from build123d import *

# Parameters (mm, degrees)
SKETCH1_R           = 1.85
SKETCH1_R_2         = 4
BOSS_EXTRUDE1_DEPTH = 2
CUT_EXTRUDE1_DEPTH  = 3


with BuildPart() as part:
    # Sketch1 → Boss-Extrude1 (new body)
    with BuildSketch(Plane(origin=(0, 0, 0), x_dir=(1, 0, 0), z_dir=(0, 1, 0))):
        with BuildLine():
            Line((39.272536472, 22.976935119), (-24.727463528, 22.976935119))
            ThreePointArc((-24.727463528, 22.976935119), (-38.227463528, 9.476935119), (-24.727463528, -4.023064881))
            Line((-24.727463528, -4.023064881), (39.272536472, -4.023064881))
            ThreePointArc((39.272536472, -4.023064881), (52.772536472, 9.476935119), (39.272536472, 22.976935119))
        make_face()
        with Locations((-24.727463528, 17.476935119)):
            Circle(SKETCH1_R, mode=Mode.SUBTRACT)
        with Locations((-24.727463528, 9.476935119)):
            Circle(SKETCH1_R_2, mode=Mode.SUBTRACT)
        with Locations((-32.727463528, 9.476935119)):
            Circle(SKETCH1_R, mode=Mode.SUBTRACT)
        with Locations((-24.727463528, 1.476935119)):
            Circle(SKETCH1_R, mode=Mode.SUBTRACT)
        with Locations((-16.727463528, 9.476935119)):
            Circle(SKETCH1_R, mode=Mode.SUBTRACT)
        with Locations((39.272536472, 17.476935119)):
            Circle(SKETCH1_R, mode=Mode.SUBTRACT)
        with Locations((39.272536472, 9.476935119)):
            Circle(SKETCH1_R_2, mode=Mode.SUBTRACT)
        with Locations((31.272536472, 9.476935119)):
            Circle(SKETCH1_R, mode=Mode.SUBTRACT)
        with Locations((47.272536472, 9.476935119)):
            Circle(SKETCH1_R, mode=Mode.SUBTRACT)
        with Locations((39.272536472, 1.476935119)):
            Circle(SKETCH1_R, mode=Mode.SUBTRACT)
    extrude(amount=BOSS_EXTRUDE1_DEPTH)

    # Sketch2 → Cut-Extrude1 (cut, through all)
    with BuildSketch(Plane(origin=(0, 2, 0), x_dir=(1, 0, 0), z_dir=(0, 1, 0))):
        with BuildLine():
            Line((-23.067485442, 22.976935119), (42.777422328, 34.888708749))
            Line((42.777422328, 34.888708749), (45.278061915, 21.567578781))
            ThreePointArc((45.278061915, 21.567578781), (10.860216356, 10.387702722), (-23.067485442, 22.976935119))
        make_face()
        with BuildLine():
            Line((48.61621824, 19.220938968), (77.215135597, 13.399575669))
            Line((77.215135597, 13.399575669), (46.358944508, -30.129693903))
            Line((46.358944508, -30.129693903), (-23.067485442, -4.023064881))
            ThreePointArc((-23.067485442, -4.023064881), (14.611544165, 1.933144375), (48.61621824, 19.220938968))
        make_face()
    extrude(amount=-CUT_EXTRUDE1_DEPTH, mode=Mode.SUBTRACT)


solid = part.part
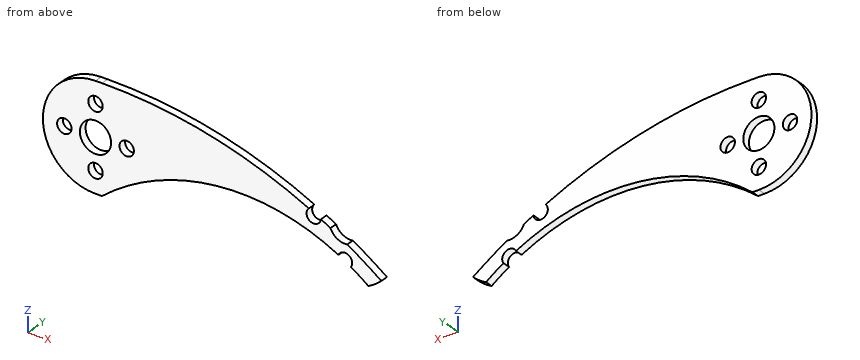
Can you work these out from the model? Positions are in its coordinate system, mm. Give positions to 0.01 mm unless a question says otherwise; leave off trailing zeros. Write each loop counter-clockwise with the first axis right and the second up, starting at its lowest first coordinate (ties: lowest second). Pieces come first, ordered by that corner, then holes. Notation, with made-up numbers: (17, -8) -> (21, -8) arc R22 cw to (21, 6) -> close; hole circle Ø8 at (62.25, -33.5). An arc over 180 degrees is marked (long way). Answer as a JSON object with one key per item and string values. Group by question number.
Item 1: Please list where these lines run through material, in increasing order: line 1 (Z direction, x = -24.5, y = 1.55); line 2 (X direction, y = 1.2, z = -18.75); line 3 (X direction, y = 1.65, z = -16.5). Write a range as [from, to].
Item 2: Suppose I cut it at A-A (y = 0.4). Please give me the cut outline in (x, z), plus the area to 3 significant figures.
Item 3: Suppose I cut it at C-C (x = 38.5). Please give me the cut outline in (y, z).
Item 4: I'm going to push a flat-ended pin straight in: P1, Ø1, axis at y = 1.5, z = -19.5, coming from the -X side. Where does the tip first touch, or does it pass through?
Item 5: Suppose I cut it at B-B (z = 2.5). Please give me the cut outline in (x, y).
Findings:
{
 "1": {"line 1": "z = [-22.98, -19.31], [-15.64, -13.47], [-5.48, -3.31], [0.36, 4.02]", "line 2": "x = [-34.54, -26.07], [-23.39, -17.2], [41.19, 47.96]", "line 3": "x = [-36.26, -26.3], [-23.16, -13.25], [37.24, 37.7], [40.84, 44.7]"},
 "2": {"outline": "(-24.73, -22.98) -> (-23.07, -22.98) arc R55.08 cw to (37.6, -16.69) arc R1.85 cw (long way) to (40.81, -18.51) arc R55.08 cw to (45.28, -21.57) arc R13.5 ccw to (48.62, -19.22) arc R122.16 ccw to (39.86, -13.43) arc R4 cw to (35.56, -10.96) arc R122.16 ccw to (33.11, -9.66) arc R1.85 cw (long way) to (30.02, -8.12) arc R122.16 ccw to (-23.07, 4.02) -> (-24.73, 4.02) arc R13.5 ccw to start; hole circle Ø3.7 at (-32.73, -9.48); hole circle Ø8 at (-24.73, -9.48); hole circle Ø3.7 at (-24.73, -17.48); hole circle Ø3.7 at (-24.73, -1.48); hole circle Ø3.7 at (-16.73, -9.48)", "area": "1,010 mm²"},
 "3": {"outline": "(0, -15.8) -> (2, -15.8) -> (2, -13.4) -> (0, -13.4) -> close"},
 "4": {"P1": "stops at x = -34.3"},
 "5": {"outline": "(-30.96, 0) -> (-3.84, 0) -> (-3.84, 2) -> (-30.96, 2) -> close"}
}
